The figure shows three views and two pictorial views of one solid part (mm, origin at its lowest corner). Answer the questions. Give positions to 0.01 mm unless a question says otherwise; leave off trailing zeros. Order: outer loops, then holes, each group sorted by start corner. A loop starts at its lowest first (then second) coordinate and runs counter-clockwise, first axis right, second up. Notation, with made-up numbers: (-26.5, 48.5) - (13.5, 48.5) arc R36 cw to (13.5, 83.5) - close; hole circle Ø2 at (48, 83). An arc over 180 degrees is marked (long way). Answer as CSV lines item,"result". Start each with the question number.
1. Section A-A on x = 63.5 is taken. Give the vertices of the cut face in (y, z).
2. Section C-C on y = 183 is taken. Give the vertices of the cut face in (x, z).
3. Flat-ended cylindrical pins translate along their axes: pin 1 (4.5 mm diameter, centred on x = 95.25, y = 196.85, fed in from +Z); pin 2 (2 mm diameter, centred on x = 70.5, z = 7, fed in from -Y). Find the tip coordinate at first contact, or state that the pin passes through.
4. Consider line 1 along Y through (x, z) = (31.75, 7); line 2 along X through (y, z) = (158.75, 5); line 3 along Y through (x, z) = (93, 0.5). Determine where each line is inside the solid, lowest interval first. Write a range as [from, to].
5. Section B-B on z = 2.25 is taken. Count the separate pieces of the cut face and the enclosed holes in it, and give its area (3 significant figures).
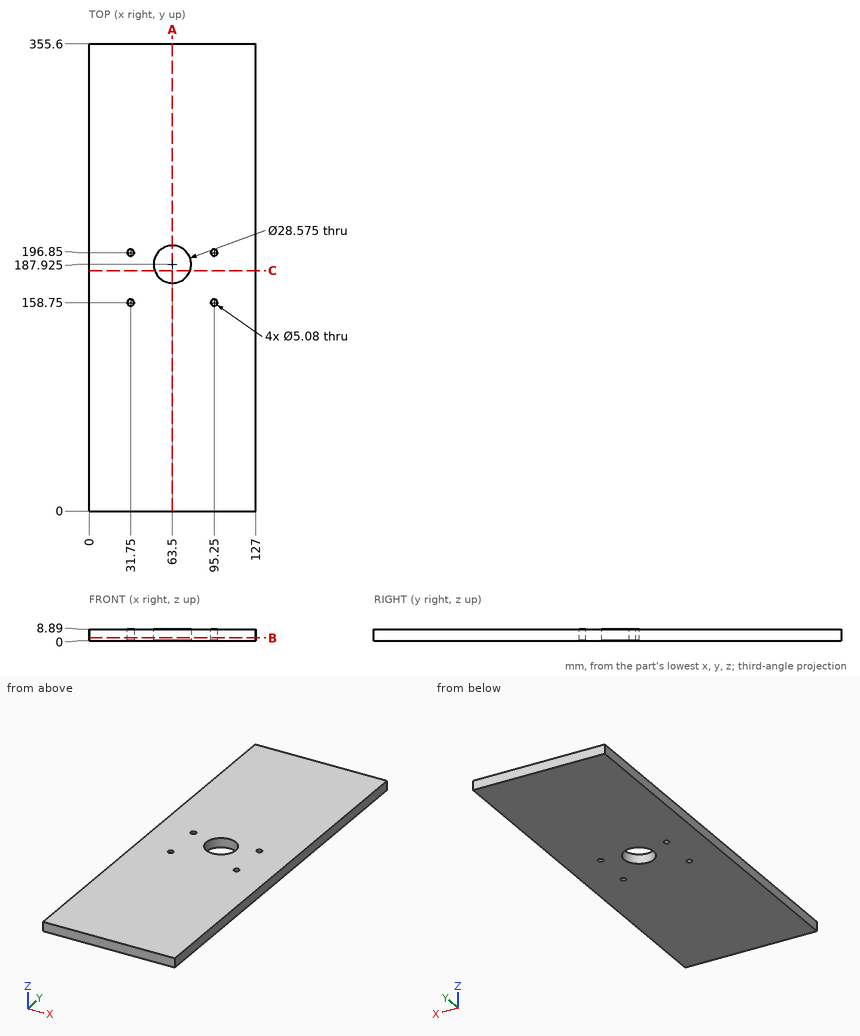
Checks:
1,outline,"(0, 0) - (173.64, 0) - (173.64, 8.89) - (0, 8.89) - close; (202.21, 0) - (355.6, 0) - (355.6, 8.89) - (202.21, 8.89) - close"
2,outline,"(0, 0) - (50.09, 0) - (50.09, 8.89) - (0, 8.89) - close; (76.91, 0) - (127, 0) - (127, 8.89) - (76.91, 8.89) - close"
3,pin 1,"passes through"
3,pin 2,"stops at y = 0"
4,line 1,"y = [0, 156.21], [161.29, 194.31], [199.39, 355.6]"
4,line 2,"x = [0, 29.21], [34.29, 92.71], [97.79, 127]"
4,line 3,"y = [0, 157.57], [159.93, 195.67], [198.03, 355.6]"
5,separate pieces,"1"
5,enclosed holes,"5"
5,area,"44,400 mm²"
